Study the drawing (mm; zero at the part's minimum x, y, z) and answer. A direction names the side the tool comes from. Give positions to 0.01 mm unless a question says otherwise; leave off trailing zeros. Loops run counter-clockwise (first coordinate to the right, second up) from the corner with the lowest first, then second, coordinate; pieces in that order, holes last. Notation, with made-up numbers: M 37,39.25 L 82,39.25 A28 cw 82,75.25 Z; hole C 62.5,40 d11. An arc over 180 degrees is marked long. Use one line per item in the form item = value. Start each with the question number.
1. Straight lines are drawn through the part: line 1 (Z direction, x = 4.5, y = 1.6); line 2 (Z direction, x = 3.75, y = 5); line 3 (X direction, y = 1.75, z = 5.5). For each, find the intervals that lie inside material, in ascending order. Write a range as from..to.
2. Each of these flat-tipped pins is pushed along its axis until it touches: pin 1 Ø2.5 at (y, z) = (2, 5) entering from +X; pin 2 Ø3 at (x, y) = (3.5, 3) entering from -Z; pin 3 Ø0.6 at (x, y) = (6.5, 5.5) entering from +Z. Where does it stop, or does it pass through?
3. The part is cut by section B-B (x = 3.5). Write down the section's boundary in (y, z), and give its area (3 significant figures).
4. The part is cut by section C-C (z = 6.5). Write down the section's boundary in (x, y), and give its area (3 significant figures).
5. For the marked faces 4, 5, 6 and 7, determine the directions among +Z, -Z, +X, -X, +Y, -Y from which every point of the face is accessible in a straight line to the end or side of a thin tool.
6. The part is cut by section D-D (y = 0.9). Write down the section's boundary in (x, z), and give its area (3 significant figures).
7. The part is cut by section A-A (y = 3). Write down the section's boundary in (x, z).
8. The mould has two halves that part along X. Classify the marked faces 1, 2 and 3: released by +X, released by -X, zero draft, split by the parting line, or undercut.
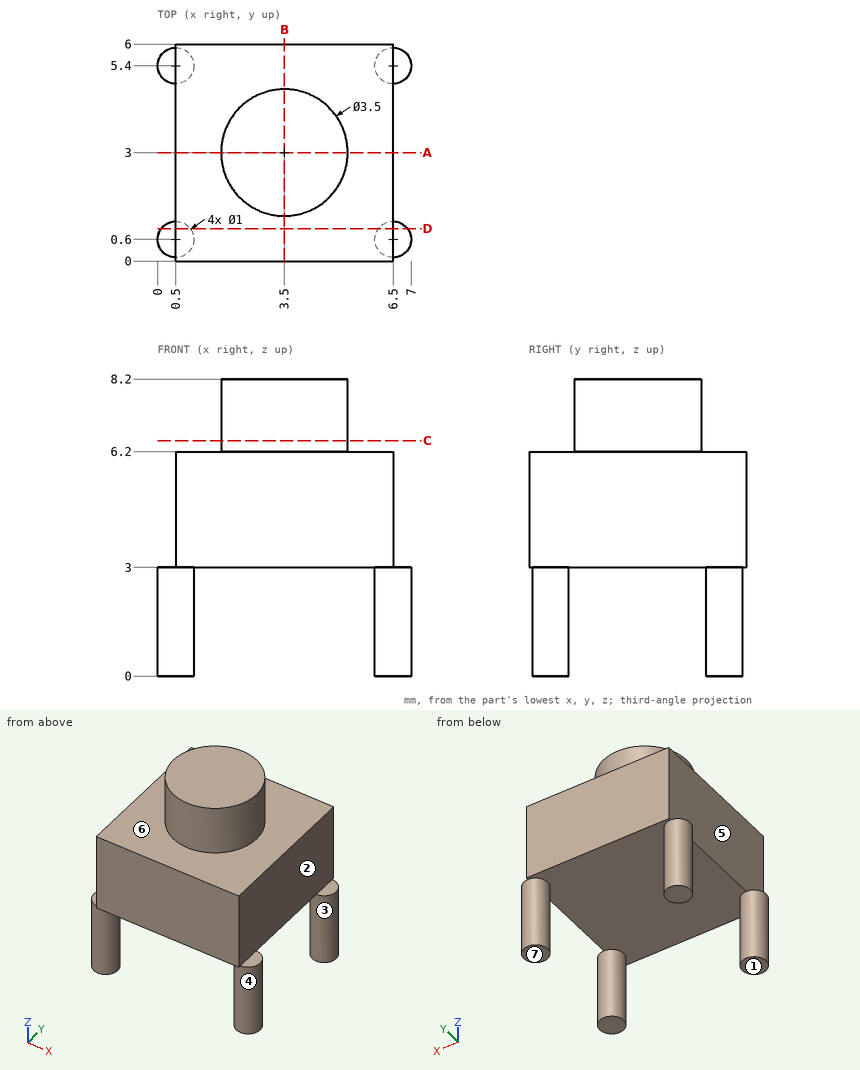
Derived:
q1.line_1 = 3..8.2
q1.line_2 = 3..6.2
q1.line_3 = 0.5..6.5
q2.pin_1 = 6.5
q2.pin_2 = 3
q2.pin_3 = 6.2
q3.outline = M 0,3 L 6,3 L 6,6.2 L 4.75,6.2 L 4.75,8.2 L 1.25,8.2 L 1.25,6.2 L 0,6.2 Z
q3.area = 26.2 mm2
q4.outline = C 3.5,3 d3.5
q4.area = 9.62 mm2
q5.face_4 = -Z
q5.face_5 = +Z, -X, +Y, -Y
q5.face_6 = +Z
q5.face_7 = -Z, +X, -X, +Y, -Y
q6.outline = M 0.1,0 L 0.9,0 L 0.9,3 L 6.1,3 L 6.1,0 L 6.9,0 L 6.9,3 L 6.5,3 L 6.5,6.2 L 0.5,6.2 L 0.5,3 L 0.1,3 Z
q6.area = 24.0 mm2
q7.outline = M 0.5,3 L 6.5,3 L 6.5,6.2 L 5.25,6.2 L 5.25,8.2 L 1.75,8.2 L 1.75,6.2 L 0.5,6.2 Z
q8.face_1 = zero draft
q8.face_2 = released by +X
q8.face_3 = undercut
